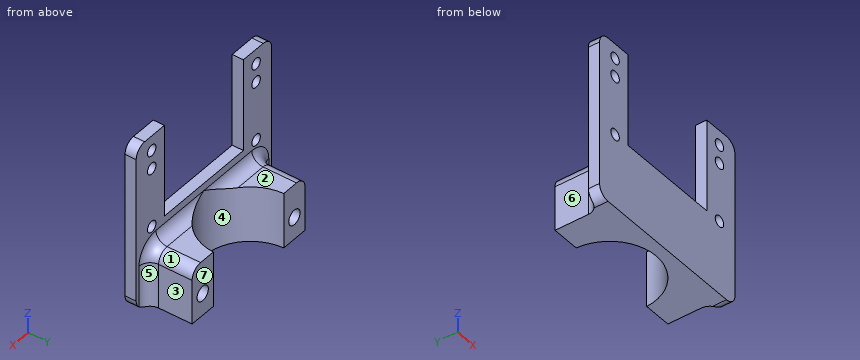
from build123d import *

# Parameters (mm, degrees)
SKETCH1_R           = 1.5
BOSS_EXTRUDE1_DEPTH = 3
SKETCH4_W           = 40
SKETCH4_H           = 15
BOSS_EXTRUDE2_DEPTH = 15
FILLET5_R           = 3
SKETCH5_R           = 12.5
CUT_EXTRUDE1_DEPTH  = 54.160135485
SKETCH6_R           = 2
CUT_EXTRUDE2_DEPTH  = 5


with BuildPart() as part:
    # Sketch1 → Boss-Extrude1 (new body)
    with BuildSketch(Plane(origin=(0, 0, 0), x_dir=(1, 0, 0), z_dir=(0, 1, 0))):
        with BuildLine():
            Line((21, 22.5), (-21, 22.5))
            ThreePointArc((-21, 22.5), (-23.121320344, 21.621320344), (-24, 19.5))
            Line((-24, 19.5), (-24, -19.5))
            ThreePointArc((-24, -19.5), (-23.121320344, -21.621320344), (-21, -22.5))
            Line((-21, -22.5), (-14, -22.5))
            Line((-14, -22.5), (-14, 2.5))
            Line((-14, 2.5), (14, 2.5))
            Line((14, 2.5), (14, -22.5))
            Line((14, -22.5), (21, -22.5))
            ThreePointArc((21, -22.5), (23.121320344, -21.621320344), (24, -19.5))
            Line((24, -19.5), (24, 19.5))
            ThreePointArc((24, 19.5), (23.121320344, 21.621320344), (21, 22.5))
        make_face()
        with Locations(Location((-18.5, -18.5, 0), (0, 0, 270))):
            Circle(SKETCH1_R, mode=Mode.SUBTRACT)
        with Locations(Location((-18.5, -13.5, 0), (0, 0, 270))):
            Circle(SKETCH1_R, mode=Mode.SUBTRACT)
        with Locations(Location((18.5, -18.5, 0), (0, 0, 270))):
            Circle(SKETCH1_R, mode=Mode.SUBTRACT)
        with Locations(Location((18.5, -13.5, 0), (0, 0, 270))):
            Circle(SKETCH1_R, mode=Mode.SUBTRACT)
        with Locations(Location((-18.5, 2.5, 0), (0, 0, 270))):
            Circle(SKETCH1_R, mode=Mode.SUBTRACT)
        with Locations(Location((18.5, 2.5, 0), (0, 0, 270))):
            Circle(SKETCH1_R, mode=Mode.SUBTRACT)
    extrude(amount=BOSS_EXTRUDE1_DEPTH)

    # Sketch4 → Boss-Extrude2 (add)
    with BuildSketch(Plane(origin=(0, 0, -22.5), x_dir=(-1, 0, 0), z_dir=(0, 0, -1))):
        with Locations((0, 7.5)):
            Rectangle(SKETCH4_W, SKETCH4_H)
    extrude(amount=-BOSS_EXTRUDE2_DEPTH)

    # Fillet5
    fillet5_edges = [part.edges().sort_by_distance(p)[0] for p in [
        (20, 3, -15),
        (-20, 3, -15),
        (0, 3, -7.5),
        (20, 9, -7.5),
        (-20, 9, -7.5),
    ]]
    fillet(fillet5_edges, radius=FILLET5_R)

    # Sketch5 → Cut-Extrude1 (cut, through all)
    with BuildSketch(Plane(origin=(0, 0, -22.5), x_dir=(-1, 0, 0), z_dir=(0, 0, -1))):
        with Locations((0, 15.5)):
            Circle(SKETCH5_R)
    extrude(amount=-CUT_EXTRUDE1_DEPTH, mode=Mode.SUBTRACT)

    # Sketch6 → Cut-Extrude2 (cut)
    with BuildSketch(Plane(origin=(0, 15, 0), x_dir=(1, 0, 0), z_dir=(0, 1, 0))):
        with Locations(Location((-16.244997998, 16.5, 0), (0, 0, 270))):
            Circle(SKETCH6_R)
        with Locations(Location((16.244997998, 16.5, 0), (0, 0, 90))):
            Circle(SKETCH6_R)
    extrude(amount=-CUT_EXTRUDE2_DEPTH, mode=Mode.SUBTRACT)


solid = part.part
Could you check a few things on this model? Use its own coordinates, in mm. Face numbers are marked on the shaded views. A direction names the side the tool comes from. Round coordinates to 2 decimals unless told otherwise and drop trailing zeros. Write each loop counter-clockwise with the first axis right and the second up, starting at its lowest first coordinate (ties: lowest second). Pieces come first, ordered by that corner, then holes. Notation, with made-up numbers: (-19, -27.5) - (11, -27.5) arc R10 ccw to (11, -12.5) - close; hole circle Ø8 at (3, 43.25). An arc over 180 degrees is marked (long way). Put each result on its own line as item: value. Start each with the question number.
(1) I want a section at A-A, the plane z = 3.5. Please give me the cut outline in (x, y).
(2) For the marked faces 1, 2 and 3, which set-ups out of +Z, -Z, +X, -X, +Y, -Y let a thin tool reach every point of the face, with its end or its side?
(3) I want a section at B-B, the plane y = 13.5. Please give me the cut outline in (x, z) (3 decimals).
(4) I want a section at D-D, the plane z = -16.5. Please give me the cut outline in (x, y) (3 decimals), plus the area to 3 significant figures.
(5) Will these pins go through, and if not, where does the flat tip stop? pin 1 (2.5 mm diameter, centred on x = -18.5, z = 13.5, fed in from -Y); pin 2 (3 mm diameter, centred on x = 19, z = 13.5, fed in from +Y); pin 3 (1.5 mm diameter, centred on x = -2.5, y = 1.5, fed in from +Z); pin 4 (2 mm diameter, centred on x = -17, z = -16, fed in from +Y).
(6) I need wall thicknesses on probe 1 along X at (y, z) = (1.6, 18.5); probe 2 along X at (y, z) = (14, -17); probe 3 along X at (y, z) = (1.75, -3). Which ranges of each line are inside material? Lowest first, please.
(7) Thinking about a two-plate mould opening in X: for the marked faces 4, 5, 6 and 7, which applies, released by +X, released by -X, zero draft, split by the parting line, or undercut?
(8) I want a section at C-C, the plane z = 13.5. Please give me the cut outline in (x, y), plus the area to 3 significant figures.
Here are the results:
1. outline: (-24, 0) - (-14, 0) - (-14, 3) - (-24, 3) - close; (14, 0) - (24, 0) - (24, 3) - (14, 3) - close
2. face 1: +Z, +X, +Y
2. face 2: +Z, +X, -X, +Y
2. face 3: +Z, -Z, +X, +Y
3. outline: (-20, -22.5) - (-12.339, -22.5) - (-12.339, -7.5) - (-17, -7.5) arc R3 ccw to (-20, -10.5) - close; (12.339, -22.5) - (20, -22.5) - (20, -10.5) arc R3 ccw to (17, -7.5) - (12.339, -7.5) - close; hole circle Ø4 at (-16.245, -16.5); hole circle Ø4 at (16.245, -16.5)
4. outline: (-24, 0) - (24, 0) - (24, 3) - (23, 3) arc R3 cw to (20, 6) - (20, 15) - (18.245, 15) - (18.245, 10) - (14.245, 10) - (14.245, 15) - (12.49, 15) arc R12.5 cw to (-12.49, 15) - (-14.245, 15) - (-14.245, 10) - (-18.245, 10) - (-18.245, 15) - (-20, 15) - (-20, 6) arc R3 cw to (-23, 3) - (-24, 3) - close
4. area: 355 mm^2
5. pin 1: passes through
5. pin 2: stops at y = 3
5. pin 3: stops at z = -2.5
5. pin 4: stops at y = 10
6. probe 1: x = -24 to -20, -17 to -14, 14 to 17, 20 to 24
6. probe 2: x = -20 to -18.18, -14.31 to -12.41, 12.41 to 14.31, 18.18 to 20
6. probe 3: x = -24 to -19.91, -17.09 to 17.09, 19.91 to 24
7. face 4: undercut
7. face 5: released by +X
7. face 6: released by -X
7. face 7: zero draft
8. outline: (-24, 0) - (-20, 0) - (-20, 3) - (-24, 3) - close; (-17, 0) - (-14, 0) - (-14, 3) - (-17, 3) - close; (14, 0) - (17, 0) - (17, 3) - (14, 3) - close; (20, 0) - (24, 0) - (24, 3) - (20, 3) - close
8. area: 42.0 mm^2
